from build123d import *

# Parameters (mm, degrees)
BOSS_EXTRUDE1_DEPTH = 20
CUT_EXTRUDE21_DEPTH = 45
CUT_EXTRUDE23_DEPTH = 444
SKETCH9_R           = 3.25
SKETCH9_R_2         = 3.15
CUT_EXTRUDE24_DEPTH = 45
CUT_EXTRUDE26_DEPTH = 444
CUT_EXTRUDE27_DEPTH = 45


with BuildPart() as part:
    # Sketch1 → Boss-Extrude1 (new body)
    with BuildSketch(Plane(origin=(0, 0, 0), x_dir=(1, 0, 0), z_dir=(0, 1, 0))):
        Polygon((-22.5, 144), (-22.5, 94), (-22.5, 74), (-17.5, 74), (-17.5, 94), (-12.5, 94), (-12.5, 74), (-7.5, 74), (-7.5, 94), (-2.5, 94), (2.5, 94), (7.5, 94), (7.5, 74), (12.5, 74), (12.5, 94), (17.5, 94), (17.5, 74), (22.5, 74), (22.5, 94), (22.5, 144), (22.5, 164), (17.5, 164), (17.5, 144), (12.5, 144), (12.5, 164), (7.5, 164), (7.5, 144), (2.5, 144), (-2.5, 144), (-7.5, 144), (-7.5, 164), (-12.5, 164), (-12.5, 144), (-17.5, 144), (-17.5, 164), (-22.5, 164), align=None)
    extrude(amount=BOSS_EXTRUDE1_DEPTH)

    # Sketch7 → Cut-Extrude21 (cut)
    with BuildSketch(Plane(origin=(22.5, 0, 0), x_dir=(0, 0, -1), z_dir=(1, 0, 0))):
        with BuildLine():
            ThreePointArc((73.999126156, 8.5), (76.488718516, 14.51040764), (82.499126156, 17))
            Line((82.499126156, 17), (93.999126156, 17))
            Line((93.999126156, 17), (93.999126156, 20))
            Line((93.999126156, 20), (82.499126156, 20))
            Line((82.499126156, 20), (73.999126156, 20))
            Line((73.999126156, 20), (73.999126156, 17))
            Line((73.999126156, 17), (73.999126156, 8.5))
        make_face()
        with BuildLine():
            ThreePointArc((82.499126156, 0), (76.488718516, 2.48959236), (73.999126156, 8.5))
            Line((73.999126156, 8.5), (73.999126156, 0))
            Line((73.999126156, 0), (82.499126156, 0))
        make_face()
        with BuildLine():
            Line((155.499126156, 20), (143.999126156, 20))
            Line((143.999126156, 20), (143.999126156, 17))
            Line((143.999126156, 17), (155.499126156, 17))
            ThreePointArc((155.499126156, 17), (163.999126156, 8.5), (155.499126156, 0))
            Line((155.499126156, 0), (163.999126156, 0))
            Line((163.999126156, 0), (164, 0))
            Line((164, 0), (164, 20))
            Line((164, 20), (163.999126156, 20))
            Line((163.999126156, 20), (155.499126156, 20))
        make_face()
    extrude(amount=-CUT_EXTRUDE21_DEPTH, mode=Mode.SUBTRACT)

    # Sketch2 → Cut-Extrude23 (cut)
    with BuildSketch(Plane.XY.offset(50)):
        with BuildLine():
            Line((-22.5, 20), (22.5, 20))
            Line((22.5, 20), (22.5, 16))
            ThreePointArc((22.5, 16), (20.832845478, 17.631987193), (18.5, 17.607120136))
            ThreePointArc((18.5, 17.607120136), (0, 13.071891388), (-18.5, 17.607120136))
            ThreePointArc((-18.5, 17.607120136), (-20.832845478, 17.631987193), (-22.5, 16))
            Line((-22.5, 16), (-22.5, 20))
        make_face()
    extrude(amount=-CUT_EXTRUDE23_DEPTH, mode=Mode.SUBTRACT)

    # Sketch9 → Cut-Extrude24 (cut)
    with BuildSketch(Plane(origin=(22.5, 0, 0), x_dir=(0, 0, -1), z_dir=(1, 0, 0))):
        with Locations((153.999563078, 8.466039352)):
            Circle(SKETCH9_R)
        with Locations((84, 8.405099657)):
            Circle(SKETCH9_R)
        with Locations((178, 8.5)):
            Circle(SKETCH9_R_2)
        with Locations((60, 8.5)):
            Circle(SKETCH9_R_2)
    extrude(amount=-CUT_EXTRUDE24_DEPTH, mode=Mode.SUBTRACT)

    # Sketch12 → Cut-Extrude26 (cut)
    with BuildSketch(Plane.XY.offset(50)):
        Polygon((-1, 3.35), (-1, 6.55), (0, 6.55), (1, 6.55), (1, 3.35), align=None)
    extrude(amount=-CUT_EXTRUDE26_DEPTH, mode=Mode.SUBTRACT)

    # Sketch13 → Cut-Extrude27 (cut)
    with BuildSketch(Plane(origin=(22.5, 0, 0), x_dir=(0, 0, -1), z_dir=(1, 0, 0))):
        Polygon((118.999126156, 8), (131.699126156, 8), (131.699126156, 10), (106.299126156, 10), (106.299126156, 8), align=None)
    extrude(amount=-CUT_EXTRUDE27_DEPTH, mode=Mode.SUBTRACT)


solid = part.part
Could you check a few things on this model? Use its own coordinates, in mm. A direction names the side the tool comes from. Give positions to 0.01 mm unless a question says otherwise; leave off trailing zeros. Write each loop counter-clockwise with the first axis right and the second up, starting at its lowest first coordinate (ties: lowest second). Pieces come first, ordered by that corner, then holes. Notation, with made-up numbers: (18, 52) - (41, 52) arc R17 ccw to (41, 81) - close; hole circle Ø11 at (-24.5, -35.75). An arc over 180 degrees is marked (long way). Use CSV: the item, a comma, the result in double quotes. Start each with the question number.
Item 1: For faces 1 (the face through (-1, 5, -119)), 2 (the face through (-20, 17, -88)), 3 (the face through (0, 10, -119)), 4 (the face through (0.269, 13.073, -118.395)), 5 (the face through (20, 17, -150)), which set-ups out of +Z, -Z, +X, -X, +Y, -Y let a thin tool reach every point of the face, with its end or its side?
Item 2: If we mould it in two halves opening along X, with no side actions, what happens to faces 6 (the face through (-22.5, 6, -120)), 7 (the face through (-19.97, 9.44, -157.1)), 8 (the face through (0, 6.55, -119))? For each: pulls with the +X half, pulls with the -X half, needs draft (parallel to the pull), parting line crosses it, or undercut.
Item 3: I want a section at B-B, the plane z = -129. Please give me the cut outline in (x, y).
Item 4: I want a section at D-D, the plane x = -4.5. Please give me the cut outline in (y, z), then the cut area to 3 significant figures.
Item 5: I want a section at A-A, the plane z = -84. Give the number of separate pieces and of enclosed holes in the cut face, then the cut area to 3 significant figures.
Item 6: I'm going to push flat-ended pins straight in: pin 1 (10.5 mm diameter, centred on y = 8.47, z = -154, fed in from +X); pin 2 (10 mm diameter, centred on x = -9, y = 2, fed in from +Z); pin 3 (6 mm diameter, centred on x = -1, y = 5.5, fed in from -Z); pin 4 (4 mm diameter, centred on x = -3.5, y = 3.5, fed in from +Z). Where does each tip first touch, or does it pass through?
Item 7: If I drill on line 1 along Y through (x, z) = (0.5, -120.5); line 2 along X through (y, z) = (9, -77.5); line 3 along Z through (x, y) = (-9, 8.75), over which ranges is the centre line in solid material (lowest first)?
Item 8: I want a section at C-C, the plane y = 1. Please give me the cut outline in (x, z).
Findings:
1,face 1,"+Z, -Z"
1,face 2,"+Z, +X, -X, +Y"
1,face 3,"+X, -X"
1,face 4,"+Z, -Z, +Y"
1,face 5,"-Z, +X, -X, +Y"
2,face 6,"pulls with the -X half"
2,face 7,"needs draft"
2,face 8,"undercut"
3,outline,"(-22.5, 0) - (22.5, 0) - (22.5, 8) - (-22.5, 8) - close; (-22.5, 10) - (22.5, 10) - (22.5, 16) arc R3.05 ccw to (18.5, 17.61) arc R40 cw to (-18.5, 17.61) arc R3.05 ccw to (-22.5, 16) - close; hole (-1, 3.35) - (1, 3.35) - (1, 6.55) - (-1, 6.55) - close"
4,outline,"(0, -144) - (13.33, -144) - (13.33, -94) - (0, -94) - close; hole (8, -131.7) - (10, -131.7) - (10, -106.3) - (8, -106.3) - close"
4,area,"615 mm2"
5,separate pieces,"8"
5,enclosed holes,"0"
5,area,"183 mm2"
6,pin 1,"stops at x = 22.5"
6,pin 2,"stops at z = -74.13"
6,pin 3,"stops at z = -144"
6,pin 4,"stops at z = -94"
7,line 1,"y = 0 to 3.35, 6.55 to 8, 10 to 13.08"
7,line 2,"x = -22.5 to -17.5, -12.5 to -7.5, 7.5 to 12.5, 17.5 to 22.5"
7,line 3,"z = -164 to -157.24, -150.76 to -131.7, -106.3 to -87.23, -80.77 to -74"
8,outline,"(-22.5, -159.5) - (-17.5, -159.5) - (-17.5, -144) - (-12.5, -144) - (-12.5, -159.5) - (-7.5, -159.5) - (-7.5, -144) - (7.5, -144) - (7.5, -159.5) - (12.5, -159.5) - (12.5, -144) - (17.5, -144) - (17.5, -159.5) - (22.5, -159.5) - (22.5, -78.5) - (17.5, -78.5) - (17.5, -94) - (12.5, -94) - (12.5, -78.5) - (7.5, -78.5) - (7.5, -94) - (-7.5, -94) - (-7.5, -78.5) - (-12.5, -78.5) - (-12.5, -94) - (-17.5, -94) - (-17.5, -78.5) - (-22.5, -78.5) - close"
